Input: part model. Units: mm. Frame: model coordinates. A direction names the side the tool comes from. Give positions to 0.01 mm unless a question says otherwise; leave off trailing zeros. Loops run counter-clockwise (first coordinate to the right, second up) from the corner with the lowest first, then second, coordinate; pieces in that order, holes last. Notation, with made-up numbers: (73.5, 9.5) -> (83.5, 9.5) arc R37 cw to (83.5, 47.5) -> close; hole circle Ø5 at (-25.5, 48). An arc over 180 degrees is marked (long way). One line per question, with ' | ' between items.
from build123d import *

# Parameters (mm, degrees)
ESQUISSE1_W                  = 220
ESQUISSE1_H                  = 150
BOSS_EXTRU_1_DEPTH           = 14.5
ENL_V_MAT_EXTRU_1_DEPTH      = 267.665052078
ENL_V_MAT_EXTRU_1_DEPTH_BACK = 267.665052078
ESQUISSE2_R                  = 2
ESQUISSE3_R                  = 4
ENL_V_MAT_EXTRU_2_DEPTH      = 4
ENL_V_MAT_EXTRU_3_DEPTH      = 267.665052078
ENL_V_MAT_EXTRU_3_DEPTH_BACK = 267.665052078
ESQUISSE4_R                  = 3.4


with BuildPart() as part:
    # Esquisse1 → Boss.-Extru.1 (new body)
    with BuildSketch(Plane.XY):
        with Locations((110, 75)):
            Rectangle(ESQUISSE1_W, ESQUISSE1_H)
    extrude(amount=BOSS_EXTRU_1_DEPTH)

    # Esquisse2 → Enlèv. mat.-Extru.1 (cut, two sides: drawn at the far end of the back side and taken through both)
    with BuildSketch(Plane.XY.offset(14.5).offset(-ENL_V_MAT_EXTRU_1_DEPTH_BACK)):
        with Locations((33, 43)):
            Circle(ESQUISSE2_R)
        with Locations((33, 17)):
            Circle(ESQUISSE2_R)
        with Locations((7, 17)):
            Circle(ESQUISSE2_R)
        with Locations((7, 43)):
            Circle(ESQUISSE2_R)
        with Locations((213, 43)):
            Circle(ESQUISSE2_R)
        with Locations((213, 17)):
            Circle(ESQUISSE2_R)
        with Locations((187, 17)):
            Circle(ESQUISSE2_R)
        with Locations((187, 43)):
            Circle(ESQUISSE2_R)
        with Locations((187, 107)):
            Circle(ESQUISSE2_R)
        with Locations((187, 133)):
            Circle(ESQUISSE2_R)
        with Locations((213, 133)):
            Circle(ESQUISSE2_R)
        with Locations((213, 107)):
            Circle(ESQUISSE2_R)
        with Locations((7, 107)):
            Circle(ESQUISSE2_R)
        with Locations((7, 133)):
            Circle(ESQUISSE2_R)
        with Locations((33, 133)):
            Circle(ESQUISSE2_R)
        with Locations((33, 107)):
            Circle(ESQUISSE2_R)
    extrude(amount=ENL_V_MAT_EXTRU_1_DEPTH + ENL_V_MAT_EXTRU_1_DEPTH_BACK, mode=Mode.SUBTRACT)

    # Esquisse3 → Enlèv. mat.-Extru.2 (cut)
    with BuildSketch(Plane.XY):
        with Locations((7, 17)):
            Circle(ESQUISSE3_R)
        with Locations((33, 17)):
            Circle(ESQUISSE3_R)
        with Locations((33, 43)):
            Circle(ESQUISSE3_R)
        with Locations((7, 43)):
            Circle(ESQUISSE3_R)
        with Locations(Location((213, 43, 0), (0, 0, 180))):
            Circle(ESQUISSE3_R)
        with Locations(Location((187, 43, 0), (0, 0, 180))):
            Circle(ESQUISSE3_R)
        with Locations(Location((187, 17, 0), (0, 0, 180))):
            Circle(ESQUISSE3_R)
        with Locations(Location((213, 17, 0), (0, 0, 180))):
            Circle(ESQUISSE3_R)
        with Locations((213, 133)):
            Circle(ESQUISSE3_R)
        with Locations((187, 133)):
            Circle(ESQUISSE3_R)
        with Locations((187, 107)):
            Circle(ESQUISSE3_R)
        with Locations((213, 107)):
            Circle(ESQUISSE3_R)
        with Locations(Location((7, 107, 0), (0, 0, 180))):
            Circle(ESQUISSE3_R)
        with Locations(Location((33, 107, 0), (0, 0, 180))):
            Circle(ESQUISSE3_R)
        with Locations(Location((33, 133, 0), (0, 0, 180))):
            Circle(ESQUISSE3_R)
        with Locations(Location((7, 133, 0), (0, 0, 180))):
            Circle(ESQUISSE3_R)
    extrude(amount=ENL_V_MAT_EXTRU_2_DEPTH, mode=Mode.SUBTRACT)

    # Esquisse4 → Enlèv. mat.-Extru.3 (cut, two sides: drawn at the far end of the back side and taken through both)
    with BuildSketch(Plane(origin=(0, 0, 0), x_dir=(-1, 0, 0), z_dir=(0, 0, -1)).offset(-ENL_V_MAT_EXTRU_3_DEPTH_BACK)):
        with Locations((-165.5, 130)):
            Circle(ESQUISSE4_R)
        with Locations((-165.5, 105)):
            Circle(ESQUISSE4_R)
        with Locations((-165.5, 80)):
            Circle(ESQUISSE4_R)
        with Locations((-54.5, 80)):
            Circle(ESQUISSE4_R)
        with Locations((-54.5, 105)):
            Circle(ESQUISSE4_R)
        with Locations((-54.5, 130)):
            Circle(ESQUISSE4_R)
    extrude(amount=ENL_V_MAT_EXTRU_3_DEPTH + ENL_V_MAT_EXTRU_3_DEPTH_BACK, mode=Mode.SUBTRACT)


solid = part.part
1. Reachability of faces 1 (the cylindrical face through (212.479, 136.966, 1.972)), 2 (the cylindrical face through (185.526, 108.352, 9.176)) from +Z, -Z, +X, -X, +Y, -Y: full face, straight path, thin tool, end or side. Return the list, or none.
Determined:
face 1: -Z | face 2: +Z, -Z
2. Pin query (flat end, axial travel): P1, Ø6.5, axis at x = 187, y = 107, coming from the -Z side. Return the tip coordinate at first contact, or that it passes through.
Determined:
P1: stops at z = 4
3. Pull-direction query (Y, two-part tool) for faces 3 (the cylindrical face through (211.4, 41.8, 9.2)), 4 (the flat face through (108, 150, 7)), 5 (the flat face through (212, 41, 4)); classes: pulls with the +Y half, pulls with the -Y half, needs draft (parallel to the pull), parting line crosses it, or undercut.
Determined:
face 3: undercut | face 4: pulls with the +Y half | face 5: undercut
4. Ray query, line 1 along Y through (x, z) = (33, 1.05); line 2 along Y through (x, z) = (187, 8.75); line 3 along X through (y, z) = (17, 7). Return the intervals inside material, ascending. Write a range as from..to.
Determined:
line 1: y = 0..13, 21..39, 47..103, 111..129, 137..150 | line 2: y = 0..15, 19..41, 45..105, 109..131, 135..150 | line 3: x = 0..5, 9..31, 35..185, 189..211, 215..220
5. Section query A-A (y = 80). Output: boundary loops of the cut face in (x, z), then the cut area to 3 significant figures.
Determined:
outline: (0, 0) -> (51.1, 0) -> (51.1, 14.5) -> (0, 14.5) -> close; (57.9, 0) -> (162.1, 0) -> (162.1, 14.5) -> (57.9, 14.5) -> close; (168.9, 0) -> (220, 0) -> (220, 14.5) -> (168.9, 14.5) -> close | area: 2,990 mm2
